```python
from build123d import *
from OCP.BRepFilletAPI import BRepFilletAPI_MakeChamfer

# Parameters (mm, degrees)
SKETCH2_W                      = 51
SKETCH2_H                      = 51
SKETCH2_R                      = 3.25
BOSS_EXTRUDE2_DEPTH            = 7
BOSS_EXTRUDE3_DEPTH            = 115
F_6_5_6_5_DIAMETER_HOLE1_D     = 6.5
F_6_5_6_5_DIAMETER_HOLE1_DEPTH = 6
F_6_5_6_5_DIAMETER_HOLE1_TIP   = 1.952797012
F_6_5_6_5_DIAMETER_HOLE2_D     = 6.5
F_6_5_6_5_DIAMETER_HOLE2_DEPTH = 6
F_6_5_6_5_DIAMETER_HOLE2_TIP   = 1.952797012
CHAMFER1_SIZE                  = 45
CHAMFER1_SIZE2                 = 17.273881577
FILLET1_R                      = 5
FILLET2_R                      = 60
FILLET3_R                      = 5


with BuildPart() as part:
    # Sketch2 → Boss-Extrude2 (new body)
    with BuildSketch(Plane(origin=(0, 0, 0), x_dir=(1, 0, 0), z_dir=(0, 1, 0))):
        with Locations((25.5, 25.5)):
            Rectangle(SKETCH2_W, SKETCH2_H)
        with Locations(Location((36, 36, 0), (0, 0, 270))):
            Circle(SKETCH2_R, mode=Mode.SUBTRACT)
    extrude(amount=BOSS_EXTRUDE2_DEPTH)

    # Sketch3 → Boss-Extrude3 (add)
    with BuildSketch(Plane(origin=(0, 7, 0), x_dir=(1, 0, 0), z_dir=(0, 1, 0))):
        Polygon((51, 0), (0, 0), (0, 51), (6, 51), (6, 6), (51, 6), align=None)
    extrude(amount=BOSS_EXTRUDE3_DEPTH)

    # Ø6.5 (6.5) Diameter Hole1
    with Locations(Plane.XY):
        with Locations((36, 107)):
            Hole(F_6_5_6_5_DIAMETER_HOLE1_D / 2, depth=F_6_5_6_5_DIAMETER_HOLE1_DEPTH)
            with Locations((0, 0, -(F_6_5_6_5_DIAMETER_HOLE1_DEPTH + F_6_5_6_5_DIAMETER_HOLE1_TIP / 2))):  # 118° drill point
                Cone(0, F_6_5_6_5_DIAMETER_HOLE1_D / 2, F_6_5_6_5_DIAMETER_HOLE1_TIP, mode=Mode.SUBTRACT)

    # Ø6.5 (6.5) Diameter Hole2
    with Locations(Plane.ZY):
        with Locations((-36, 107)):
            Hole(F_6_5_6_5_DIAMETER_HOLE2_D / 2, depth=F_6_5_6_5_DIAMETER_HOLE2_DEPTH)
            with Locations((0, 0, -(F_6_5_6_5_DIAMETER_HOLE2_DEPTH + F_6_5_6_5_DIAMETER_HOLE2_TIP / 2))):  # 118° drill point
                Cone(0, F_6_5_6_5_DIAMETER_HOLE2_D / 2, F_6_5_6_5_DIAMETER_HOLE2_TIP, mode=Mode.SUBTRACT)

    # Chamfer1: one chamfer whose edges measure the first distance from different faces: ONE call of the kernel's chamfer builder (chamfer() names one face for all edges)
    chamfer1_edges_1 = [part.edges().sort_by_distance(p)[0] for p in [
        (28.5, 7, -6),
    ]]
    chamfer1_side_1 = [part.faces().sort_by_distance(p)[0] for p in [
        (28.451598229, 64.2257233, -6),
    ]]
    chamfer1_edges_2 = [part.edges().sort_by_distance(p)[0] for p in [
        (6, 7, -28.5),
    ]]
    chamfer1_side_2 = [part.faces().sort_by_distance(p)[0] for p in [
        (6, 64.2257233, -28.451598229),
    ]]
    chamfer1 = BRepFilletAPI_MakeChamfer(part.part.solid().wrapped)
    for e in chamfer1_edges_1:
        chamfer1.Add(CHAMFER1_SIZE, CHAMFER1_SIZE2, e.wrapped, chamfer1_side_1[0].wrapped)  # the first distance lies on this face
    for e in chamfer1_edges_2:
        chamfer1.Add(CHAMFER1_SIZE, CHAMFER1_SIZE2, e.wrapped, chamfer1_side_2[0].wrapped)  # the first distance lies on this face
    add(Compound.cast(chamfer1.Shape()), mode=Mode.REPLACE)

    # Fillet1
    fillet1_edges = [part.edges().sort_by_distance(p)[0] for p in [
        (0, 61, 0),
    ]]
    fillet(fillet1_edges, radius=FILLET1_R)

    # Fillet2
    fillet2_edges = [part.edges().sort_by_distance(p)[0] for p in [
        (28.5, 52, -6),
        (6, 52, -28.5),
    ]]
    fillet(fillet2_edges, radius=FILLET2_R)

    # Fillet3
    fillet3_edges = [part.edges().sort_by_distance(p)[0] for p in [
        (23.273881577, 7, -37.136940788),
        (37.136940788, 7, -23.273881577),
    ]]
    fillet(fillet3_edges, radius=FILLET3_R)


solid = part.part
```
Work out the finished part from the listing and answer in its coordinate system (mm). A direction names the side the tool comes from. Round coordinates to 2 decimals unless told otherwise and drop trailing zeros. Loops run counter-clockwise (first coordinate to the right, second up) from the corner with the lowest first, then second, coordinate; pieces in that order, holes last.
(1) The part is cut by section C-C, the plane y = 107. Give the vertices of the cut face in (x, z).
Computed values:
outline: (0, -51) - (6, -51) - (6, -39.25) - (0, -39.25) - close; (0, -32.75) - (6, -32.75) - (6, -6) - (32.75, -6) - (32.75, 0) - (5, 0) arc R5 ccw to (0, -5) - close; (39.25, -6) - (51, -6) - (51, 0) - (39.25, 0) - close
(2) The part is cut by section D-D, the plane z = -30. Give the vertices of the cut face in (x, y), and give its area (3 significant figures).
Computed values:
outline: (0, 0) - (51, 0) - (51, 7) - (26.71, 7) arc R5 cw to (22.04, 10.21) - (9.99, 41.62) arc R60 cw to (6, 63.12) - (6, 122) - (0, 122) - close
area: 1,450 mm2
(3) Find the intervals of material crossed by L1, parallel to Y at x = 3, z = -36; L2, parallel to X at y = 5, z = -36; L3, parallel to Z at x = 27.5, y = 82.5, in increasing order.
Computed values:
L1: y = 0 to 103.75, 110.25 to 122
L2: x = 0 to 32.75, 39.25 to 51
L3: z = -6 to 0
(4) The mould has two halves that part along X. Classify faces 3 (the cylindrical face through (36.724, 7.903, -23.844)), 4 (the flat face through (0, 60, -28)), 5 (the cylindrical face through (34.5, 104.117, -3.042)), 6 (the flat face through (6, 92, -29)): pulls with the +X half, pulls with the -X half, needs draft (parallel to the pull), parting line crosses it, or undercut.
Computed values:
face 3: needs draft
face 4: pulls with the -X half
face 5: undercut
face 6: pulls with the +X half
(5) For faces 1 (the cylindrical face through (2, 60, -1)), 2 (the cylindrical face through (28.815, 52.338, -6.977)), determine the directions among +Z, -Z, +X, -X, +Y, -Y from which every point of the face is accessible in a straight line to the end or side of a thin tool.
Computed values:
face 1: +Z, -X, +Y, -Y
face 2: -Z, +X, +Y
(6) Each of these flat-tipped pins is pushed along its axis until it touches: P1, Ø13.5, axis at y = 81, z = -37, coming from the +X side; P2, Ø6, axis at y = 51, z = -19.5, coming from the +X side; P3, Ø19.5, axis at x = 41.5, z = -35, coming from the +Y side. Where does it stop, or does it pass through?
Computed values:
P1: stops at x = 6
P2: stops at x = 7.94
P3: stops at y = 7.22
(7) The part is cut by section A-A, the plane x = 36. Give the vertices of the cut face in (y, z).
Computed values:
outline: (0, -51) - (7, -51) - (7, -39.25) - (0, -39.25) - close; (0, -32.75) - (7, -32.75) - (7, -26.71) arc R5 cw to (10.21, -22.04) - (41.62, -9.99) arc R60 cw to (63.12, -6) - (103.75, -6) - (103.75, 0) - (0, 0) - close; (110.25, -6) - (122, -6) - (122, 0) - (110.25, 0) - close
(8) The part is cut by section B-B, the plane z = -36. Give the vertices of the cut face in (x, y).
Computed values:
outline: (0, 0) - (32.75, 0) - (32.75, 7) - (26.71, 7) arc R5 cw to (22.04, 10.21) - (9.99, 41.62) arc R60 cw to (6, 63.12) - (6, 103.75) - (0, 103.75) - close; (0, 110.25) - (6, 110.25) - (6, 122) - (0, 122) - close; (39.25, 0) - (51, 0) - (51, 7) - (39.25, 7) - close
